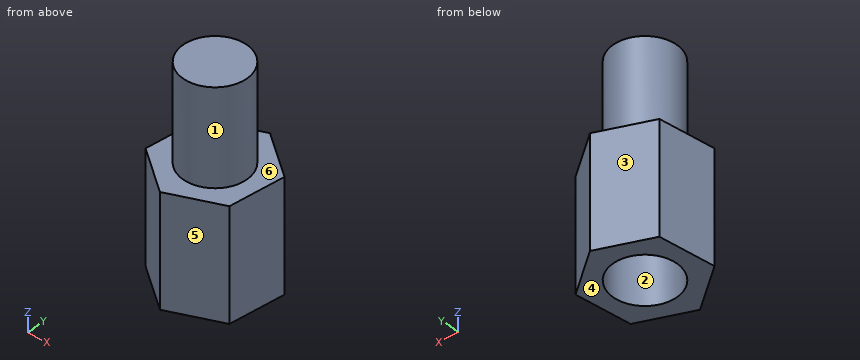
from build123d import *

# Parameters (mm, degrees)
EXTRUDE_1_DEPTH     = 7
SKETCH_2_R          = 2
EXTRUDE_2_DEPTH     = 6
SKETCH_3_R          = 2
CUT_EXTRUDE_1_DEPTH = 4


with BuildPart() as part:
    # 草图1 → 凸台-拉伸1 (new body)
    with BuildSketch(Plane.XY):
        Polygon((2.740200821, -2.119268615), (3.205440868, 1.313449215), (0.465240048, 3.43271783), (-2.740200821, 2.119268615), (-3.205440868, -1.313449215), (-0.465240048, -3.43271783), align=None)
    extrude(amount=EXTRUDE_1_DEPTH)

    # 草图2 → 凸台-拉伸2 (add)
    with BuildSketch(Plane.XY.offset(7)):
        Circle(SKETCH_2_R)
    extrude(amount=EXTRUDE_2_DEPTH)

    # 草图3 → 切除-拉伸1 (cut)
    with BuildSketch(Plane(origin=(0, 0, 0), x_dir=(-1, 0, 0), z_dir=(0, 0, -1))):
        Circle(SKETCH_3_R)
    extrude(amount=-CUT_EXTRUDE_1_DEPTH, mode=Mode.SUBTRACT)


solid = part.part
Geometry check sheet. Reference: the model listing, model coordinates, mm. Face numbers are marked on the shaded views. A direction names the side the tool comes from. Give positions to 0.01 mm unless a question says otherwise; leave off trailing zeros. Loops run counter-clockwise (first coordinate to the right, second up) from the corner with the lowest first, then second, coordinate; pieces in that order, holes last.
(1) Section check B-B on x = -1.25. Record the cut outline in (y, z).
From the geometry:
outline: (-2.83, 0) - (-1.56, 0) - (-1.56, 4) - (1.56, 4) - (1.56, 0) - (2.73, 0) - (2.73, 7) - (1.56, 7) - (1.56, 13) - (-1.56, 13) - (-1.56, 7) - (-2.83, 7) - close
(2) Depth check by flat-ended pin: pin 1 Ø2 at (y, z) = (-1, 5) entering from +X; pin 2 Ø2 at (x, y) = (2.5, -1.5) entering from -Z; pin 3 Ø1.5 at (x, z) = (1, 8.5) entering from -Y; pin 4 Ø3 at (x, y) = (-2.5, 2.5) entering from +Z. Enter the tip coordinate at first touch or a pass-through.
From the geometry:
pin 1: stops at x = 3.03
pin 2: stops at z = 0
pin 3: stops at y = -1.98
pin 4: stops at z = 7
(3) Release check for a two-part mould opening along X. For the marked faces 1, 2, 3 and 4 record: released by +X, released by -X, zero draft, split by the parting line, or undercut.
From the geometry:
face 1: split by the parting line
face 2: undercut
face 3: released by -X
face 4: zero draft
(4) Set-up check for the marked faces 5 and 6: record each of +Z, -Z, +X, -X, +Y, -Y from which the full face is reachable in a straight line by a thin tool's end or side.
From the geometry:
face 5: +Z, -Z, +X, -Y
face 6: +Z
(5) Section check A-A on z = 3.75. Record the cut outline in (x, y), then the cut area to 3 significant figures.
From the geometry:
outline: (-3.21, -1.31) - (-0.47, -3.43) - (2.74, -2.12) - (3.21, 1.31) - (0.47, 3.43) - (-2.74, 2.12) - close; hole circle Ø4 at (0, 0)
area: 18.6 mm2
(6) Thickness scan on L1, parallel to Y at x = 0, z = 1.8; L2, parallel to Z at x = 2.25, y = -1.25; L3, parallel to Y at x = -1.75, z = 2.5 (3 decimals). Record the ranges inside material, lowest first.
From the geometry:
L1: y = -3.24 to -2, 2 to 3.24
L2: z = 0 to 7
L3: y = -2.439 to -0.968, 0.968 to 2.525
(7) Section check D-D on z = 8.5. Record the cut outline in (x, y), then the cut area to 3 significant figures.
From the geometry:
outline: circle Ø4 at (0, 0)
area: 12.6 mm2
(8) Section check C-C on y = 0. Record the cut outline in (x, z).
From the geometry:
outline: (-3.03, 0) - (-2, 0) - (-2, 4) - (2, 4) - (2, 0) - (3.03, 0) - (3.03, 7) - (2, 7) - (2, 13) - (-2, 13) - (-2, 7) - (-3.03, 7) - close
